Design review of the part built by this model. Coordinates are the model's own, in mm. Face numbers are marked on the shaded views. A direction names the side the tool comes from. Give positions to 0.01 mm unless a question says otherwise; leave off trailing zeros. Order: outer loops, then holes, each group sorted by start corner. A loop starts at its lowest first (then second) coordinate and runs counter-clockwise, first axis right, second up. Notation, with made-up numbers: (40.25, -25.75) -> (90.25, -25.75) arc R17 ccw to (90.25, 7.25) -> close; hole circle Ø3 at (2.5, -13). An arc over 180 degrees is marked (long way). One line per item, written item: value. Start each with the question number.
1) For pin 1 (2 mm diameter, centred on x = 14.5, z = -4, fed in from -Y), flat-tipped, find the tip position at first contact; note if it passes through.
2) Consider section A-A (y = 0). State the section outline as (x, z) points.
3) Tool access review of the marked faces 4 and 5: name each direction out of +Z, -Z, +X, -X, +Y, -Y from which nothing blocks a thin tool from reaching the whole face with its end or side.
4) The part is to be moulded in two halves that separate along Z. For the marked faces 1, 2 and 3, say which applies: released by +Z, released by -Z, zero draft, split by the parting line, or undercut.
5) Consider section C-C (x = 15.55). State the section outline as (y, z) points, plus the area to 3 significant figures.
6) Wall thickness on line 1 along Z through (x, y) = (15.2, 0); line 2 along X through (y, z) = (5, -4.25); line 3 along Z through (x, y) = (13.9, 0): over which ranges is each line inside the solid? List them lowest first. Write a range as from..to.
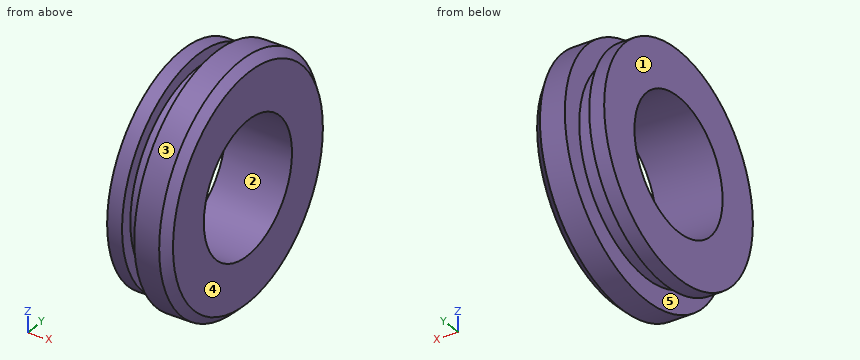
from build123d import *

# Parameters (mm, degrees)
CHAMFER_1_SIZE = 0.5


with BuildPart() as part:
    # Эскиз2 → Повернуть1 (revolve)
    with BuildSketch(Plane.XY, mode=Mode.PRIVATE) as revolve_1_sk:
        Polygon((14.5, 5.990991269), (14.5, 7.3), (16.5, 7.3), (16.5, 4), (12.5, 4), (12.5, 4.990991269), (12.5, 6.746286905), (13.39735467, 6.746286905), (13.39735467, 5.990991269), align=None)
    revolve(revolve_1_sk.sketch.rotate(Axis((0, 0, 0), (1, 0, 0)), 180), axis=Axis((0, 0, 0), (1, 0, 0)))

    # Фаска1
    chamfer_1_edges = [part.edges().sort_by_distance(p)[0] for p in [
        (16.5, 7.3, 0),
    ]]
    chamfer(chamfer_1_edges, length=CHAMFER_1_SIZE)


solid = part.part
Checked values:
1. pin 1: stops at y = -6.66
2. outline: (12.5, -6.75) -> (13.4, -6.75) -> (13.4, -5.99) -> (14.5, -5.99) -> (14.5, -7.3) -> (16, -7.3) -> (16.5, -6.8) -> (16.5, -4) -> (12.5, -4) -> close; (12.5, 4) -> (16.5, 4) -> (16.5, 6.8) -> (16, 7.3) -> (14.5, 7.3) -> (14.5, 5.99) -> (13.4, 5.99) -> (13.4, 6.75) -> (12.5, 6.75) -> close
3. face 4: +Z, -Z, +X, +Y, -Y
3. face 5: none
4. face 1: zero draft
4. face 2: undercut
4. face 3: split by the parting line
5. outline: circle Ø14.6 at (0, 0); hole circle Ø8 at (0, 0)
5. area: 117 mm^2
6. line 1: z = -7.3..-4, 4..7.3
6. line 2: x = 12.5..13.4, 14.5..16.5
6. line 3: z = -5.99..-4, 4..5.99
